```python
from build123d import *

# Parameters (mm, degrees)
BOSS_EXTRUDE1_DEPTH = 60
SKETCH4_W           = 10
SKETCH4_H           = 90
BOSS_EXTRUDE2_DEPTH = 45
SKETCH6_W           = 25
SKETCH6_H           = 10
BOSS_EXTRUDE3_DEPTH = 45
SKETCH8_W           = 10
SKETCH8_H           = 15
BOSS_EXTRUDE4_DEPTH = 90
BOSS_EXTRUDE5_DEPTH = 30
BOSS_EXTRUDE6_DEPTH = 30
CUT_EXTRUDE1_DEPTH  = 30
CUT_EXTRUDE2_DEPTH  = 25
SKETCH14_W          = 10
SKETCH14_H          = 28.5
CUT_EXTRUDE3_DEPTH  = 25
BOSS_EXTRUDE7_DEPTH = 5


with BuildPart() as part:
    # Sketch1 → Boss-Extrude1 (new body)
    with BuildSketch(Plane(origin=(0, 0, 0), x_dir=(0, 0, -1), z_dir=(1, 0, 0))):
        Polygon((0, -10), (0, 90), (10, 90), (10, 0), (25, 0), (25, -10), align=None)
    extrude(amount=BOSS_EXTRUDE1_DEPTH)

    # Sketch4 → Boss-Extrude2 (add)
    with BuildSketch(Plane(origin=(60, 0, 0), x_dir=(0, 0, -1), z_dir=(1, 0, 0))):
        with Locations((5, 45)):
            Rectangle(SKETCH4_W, SKETCH4_H)
    extrude(amount=BOSS_EXTRUDE2_DEPTH)

    # Sketch6 → Boss-Extrude3 (add)
    with BuildSketch(Plane(origin=(60, 0, 0), x_dir=(0, 0, -1), z_dir=(1, 0, 0))):
        with Locations((12.5, -5)):
            Rectangle(SKETCH6_W, SKETCH6_H)
    extrude(amount=BOSS_EXTRUDE3_DEPTH)

    # Sketch8 → Boss-Extrude4 (add)
    with BuildSketch(Plane(origin=(0, 0, 0), x_dir=(1, 0, 0), z_dir=(0, 1, 0))):
        with Locations((100, 17.5)):
            Rectangle(SKETCH8_W, SKETCH8_H)
    extrude(amount=BOSS_EXTRUDE4_DEPTH)

    # Sketch10 → Boss-Extrude5 (add)
    with BuildSketch(Plane.ZY):
        Polygon((0, -10), (0, 90), (-10, 90), (-10, 0), (-25, 0), (-25, -10), align=None)
    extrude(amount=BOSS_EXTRUDE5_DEPTH)

    # Sketch11 → Boss-Extrude6 (add)
    with BuildSketch(Plane(origin=(0, 90, 0), x_dir=(1, 0, 0), z_dir=(0, 1, 0))):
        Polygon((-30, 10), (-30, 0), (105, 0), (105, 25), (95, 25), (95, 10), align=None)
    extrude(amount=BOSS_EXTRUDE6_DEPTH)

    # Sketch12 → Cut-Extrude1 (cut)
    with BuildSketch(Plane(origin=(0, 0, -10), x_dir=(-1, 0, 0), z_dir=(0, 0, -1))):
        with BuildLine():
            Line((-25, 91.5), (30, 91.5))
            Line((30, 91.5), (30, 28.5))
            Line((30, 28.5), (-25, 28.5))
            ThreePointArc((-25, 28.5), (-56.5, 60), (-25, 91.5))
        make_face()
    extrude(amount=-CUT_EXTRUDE1_DEPTH, mode=Mode.SUBTRACT)

    # Sketch13 → Cut-Extrude2 (cut)
    with BuildSketch(Plane.ZY.offset(30)):
        Polygon((0, 28.5), (-10, 28.5), (-10, 0), (-25, 0), (-25, -10), (0, -10), align=None)
    extrude(amount=-CUT_EXTRUDE2_DEPTH, mode=Mode.SUBTRACT)

    # Sketch14 → Cut-Extrude3 (cut)
    with BuildSketch(Plane.ZY.offset(30)):
        with Locations((-5, 105.75)):
            Rectangle(SKETCH14_W, SKETCH14_H)
    extrude(amount=-CUT_EXTRUDE3_DEPTH, mode=Mode.SUBTRACT)

    # Sketch15 → Boss-Extrude7 (add)
    with BuildSketch(Plane(origin=(0, 0, -25), x_dir=(-1, 0, 0), z_dir=(0, 0, -1))):
        Polygon((5, -10), (5, 0), (-95, 0), (-95, 120), (-105, 120), (-105, -10), align=None)
    extrude(amount=BOSS_EXTRUDE7_DEPTH)


solid = part.part
```
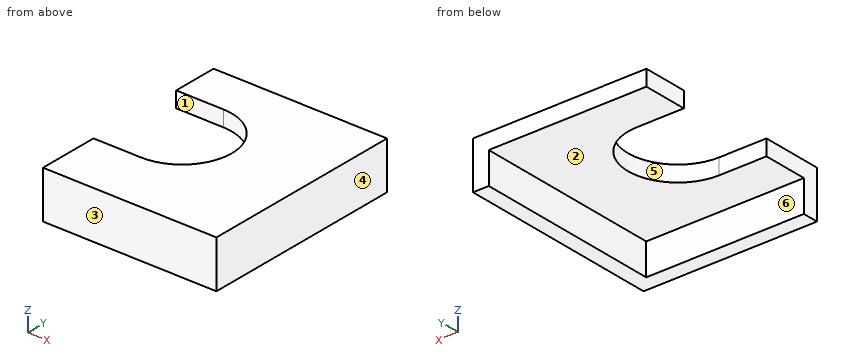
Here's how the part is built. I have some questions about the finished solid (model axes, mm). Face numbers are marked on the shaded views. A direction names the side the tool comes from. Coordinates: 2 decimals unless noted, no trailing zeros. Order: outer loops, then holes, each group sorted by start corner. A loop starts at its lowest first (then second) coordinate and runs counter-clockwise, first axis right, second up. Notation, with made-up numbers: (29, -18) -> (36, -18) arc R22 ccw to (36, 13) -> close; hole circle Ø5 at (24, -28.5). An arc over 180 degrees is marked (long way). Return JSON: item names as keys, results as strings.
1) If we section it at C-C on y = 11.5: List the corners of the cut face in (x, z) for me.
Conclusion:
{"outline": "(-5, -10) -> (95, -10) -> (95, -30) -> (105, -30) -> (105, 0) -> (-5, 0) -> close"}
2) If I drill on probe 1 along Y at (x, z) = (14.5, -1.5); probe 2 along X at (y, z) = (12, -12.25); probe 3 along Z at (x, y) = (67, 13), over which ranges is the centre line in solid material (lowest first)?
Conclusion:
{"probe 1": "y = -10 to 28.5, 91.5 to 120", "probe 2": "x = 95 to 105", "probe 3": "z = -10 to 0"}
3) If we section it at D-D on x = 83: List the corners of the cut face in (y, z) for me, plus the area to 3 significant figures.
Conclusion:
{"outline": "(-10, -30) -> (0, -30) -> (0, -10) -> (120, -10) -> (120, 0) -> (-10, 0) -> close", "area": "1,500 mm²"}
4) If we section it at A-A on z = -6.75: List the corners of the cut face in (x, y) for me, plus the area to 3 significant figures.
Conclusion:
{"outline": "(-5, -10) -> (105, -10) -> (105, 120) -> (-5, 120) -> (-5, 91.5) -> (25, 91.5) arc R31.5 cw to (25, 28.5) -> (-5, 28.5) -> close", "area": "10,900 mm²"}
5) Thinking about a two-plate mould opening in Y: for the marked faces 4, 5 and 6, which applies, +Y half, -Y half, draft (parallel to the pull), parting line (faces both ways), or undercut?
Conclusion:
{"face 4": "draft", "face 5": "undercut", "face 6": "+Y half"}
6) I'm going to push flat-ended pins straight in: P1, Ø1.5, axis at y = 13.5, z = -25, coming from the -X side; P2, Ø5, axis at x = 39.5, y = 26.5, coming from the -Z side; P3, Ø10, axis at x = 50.5, z = -18, coming from the +Y side. Where does each tip first touch, or does it pass through?
Conclusion:
{"P1": "stops at x = 95", "P2": "stops at z = -10", "P3": "stops at y = 0"}
7) If we section it at B-B on x = 36.5: List the corners of the cut face in (y, z) for me, plus the area to 3 significant figures.
Conclusion:
{"outline": "(-10, -30) -> (0, -30) -> (0, -10) -> (30.67, -10) -> (30.67, 0) -> (-10, 0) -> close; (89.33, -10) -> (120, -10) -> (120, 0) -> (89.33, 0) -> close", "area": "913 mm²"}
8) On a 3-axis mill with a long thin cutter (end or side, diameter ignored), from which of +Z, -Z, +X, -X, +Y, -Y can I reach the whole of each face in a straight line? I mean the marked faces 1, 2 and 3. Say none if no direction works.
Conclusion:
{"face 1": "+Z, -Z, -X", "face 2": "-Z, -X, +Y", "face 3": "+Z, -Z, +X, -X, -Y"}
